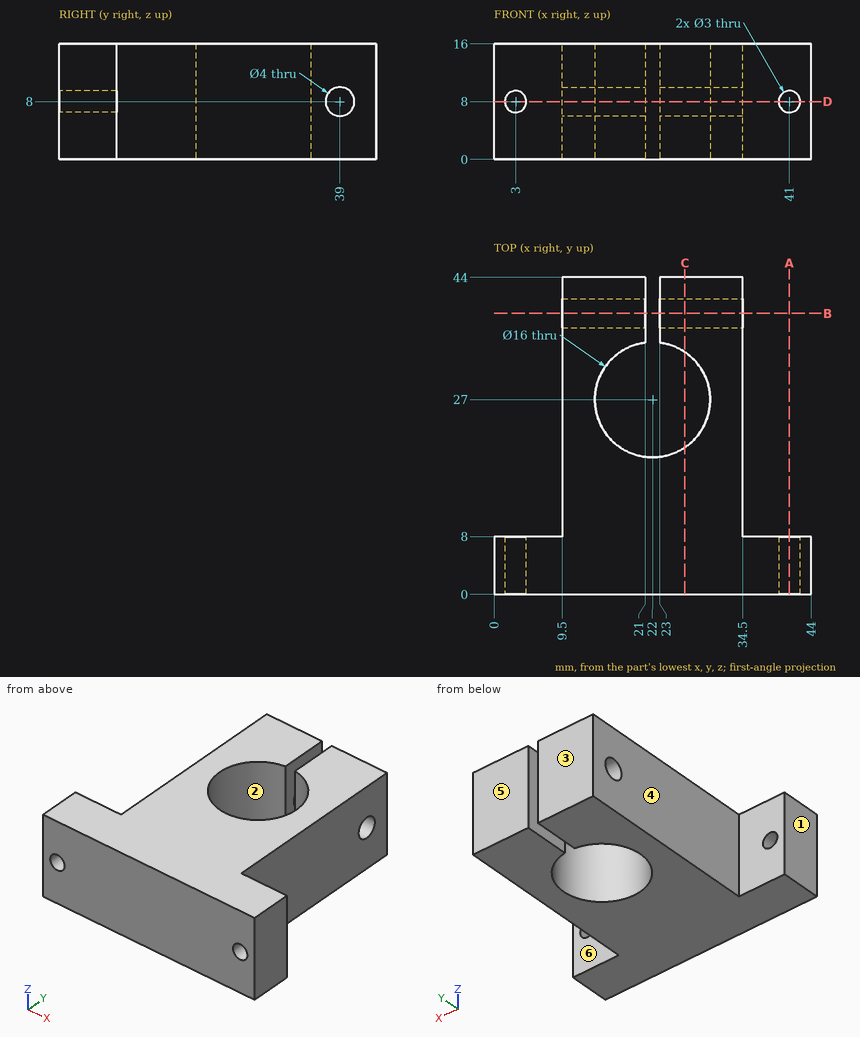
Answer from the drawing. Dimensions are ordinates in mm from the lowest x, y and z of the part. A direction names the side the tool comes from. Give positions to 0.01 mm unless a question says otherwise; leave off trailing zeros. Write each loop counter-clockwise with the first axis right and the second up, starting at its lowest first coordinate (ties: lowest second). Pieces come first, ordered by that corner, then holes. Notation, with made-up numbers: M 52,-26.5 L 110,-26.5 A14 cw 110,-10.5 Z; hole C 82,-25 d6. An arc over 180 degrees is marked long. Answer as CSV lines item,"result".
Q1. A cutting plane is placed at A-A on x = 41. Write down the section's boundary in (y, z), plus the area to 3 significant figures.
A:
outline,"M 0,0 L 8,0 L 8,6.5 L 0,6.5 Z; M 0,9.5 L 8,9.5 L 8,16 L 0,16 Z"
area,"104 mm²"
Q2. A cutting plane is placed at D-D on z = 8. Write down the section's boundary in (x, y), plus the area to 3 significant figures.
A:
outline,"M 0,0 L 1.5,0 L 1.5,8 L 0,8 Z; M 4.5,0 L 39.5,0 L 39.5,8 L 34.5,8 L 34.5,37 L 23,37 L 23,34.94 A8 cw long 21,34.94 L 21,37 L 9.5,37 L 9.5,8 L 4.5,8 Z; M 9.5,41 L 21,41 L 21,44 L 9.5,44 Z; M 23,41 L 34.5,41 L 34.5,44 L 23,44 Z; M 42.5,0 L 44,0 L 44,8 L 42.5,8 Z"
area,"893 mm²"
Q3. A cutting plane is placed at B-B on y = 39. Write down the section's boundary in (x, z), plus the area to 3 significant figures.
A:
outline,"M 9.5,0 L 21,0 L 21,6 L 9.5,6 Z; M 9.5,10 L 21,10 L 21,16 L 9.5,16 Z; M 23,0 L 34.5,0 L 34.5,6 L 23,6 Z; M 23,10 L 34.5,10 L 34.5,16 L 23,16 Z"
area,"276 mm²"
Q4. A tool of negligible diameter and unlimited length cuts with its end or side. For the marked faces 4, 5 and 6, from which of +Z, -Z, +X, -X, +Y, -Y can it reach the whole face along a straight path? Write none if from no direction.
A:
face 4,"+Z, -Z, -X, +Y"
face 5,"+Z, -Z, +X, -X, +Y"
face 6,"+Z, -Z, +X, +Y"
Q5. Given P1, Ø6.5, axis at y = 39, z = 8, coming from the -X side; P2, Ø5, axis at x = 3.5, z = 7, coming from the +Y side; P3, Ø5, axis at x = 18.5, y = 25.5, coming from the +Z side; P4, Ø4.5, axis at y = 38, z = 6, coming from the +X side, each flat-ended and moving along its own axis, determine where each tip first touches the part or whether it passes through.
A:
P1,"stops at x = 9.5"
P2,"stops at y = 8"
P3,"passes through"
P4,"stops at x = 34.5"
Q6. A cutting plane is placed at C-C on x = 26.5. Write down the section's boundary in (y, z).
A:
outline,"M 0,0 L 20.39,0 L 20.39,16 L 0,16 Z; M 33.61,0 L 44,0 L 44,16 L 33.61,16 Z; hole C 39,8 d4"
Q7. Find the intervals of material crossed by probe 1 along X at (y, z) = (27, 10); probe 2 along Y at (x, z) = (12.75, 8); probe 3 along Y at (x, z) = (16.75, 8), in increasing order. Write a range as [from, to].
A:
probe 1,"x = [9.5, 14], [30, 34.5]"
probe 2,"y = [0, 37], [41, 44]"
probe 3,"y = [0, 20.96], [33.04, 37], [41, 44]"
Q8. The mould has two halves that part along X. Classify the marked faces 1, 2 and 3: +X half, -X half, draft (parallel to the pull), parting line (faces both ways), or undercut.
A:
face 1,"-X half"
face 2,"undercut"
face 3,"draft"
